Model file for the job. Use its own axes, mm. Face numbers are marked on the shaded views. Round coordinates to 2 decimals unless told otherwise and drop trailing zeros. Write each loop counter-clockwise with the first axis right and the second up, starting at its lowest first coordinate (ties: lowest second). Pieces come first, ordered by that corner, then holes. Notation, with made-up numbers: (-40, 71.5) - (-19, 71.5) arc R10 cw to (-19, 75.5) - close; hole circle Ø7 at (66, 28). An arc over 180 degrees is marked (long way). One line per item, written item: value.
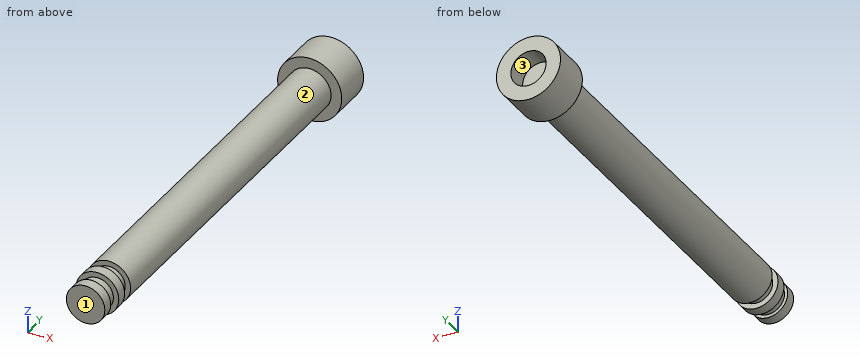
from build123d import *

# Parameters (mm, degrees)
SKETCH1_R           = 3
BOSS_EXTRUDE1_DEPTH = 3.7
SKETCH1_3_R         = 1.6
BOSS_EXTRUDE2_DEPTH = 1
SKETCH5_R           = 1.5
BOSS_EXTRUDE3_DEPTH = 35
SKETCH6_R           = 2
BOSS_EXTRUDE4_DEPTH = 1
SKETCH8_R           = 1.5
BOSS_EXTRUDE5_DEPTH = 2
SKETCH10_R          = 1.8
BOSS_EXTRUDE6_DEPTH = 1
SKETCH12_R          = 1.65
CUT_EXTRUDE1_DEPTH  = 2
SKETCH13_R          = 2
BOSS_EXTRUDE7_DEPTH = 34


with BuildPart() as part:
    # Sketch1 → Boss-Extrude1 (new body)
    with BuildSketch(Plane(origin=(0, 0, 0), x_dir=(1, 0, 0), z_dir=(0, 1, 0))):
        with Locations((-0.522013312, 0.511138034)):
            Circle(SKETCH1_R)
    extrude(amount=BOSS_EXTRUDE1_DEPTH)

    # Sketch1<3> → Boss-Extrude2 (add)
    with BuildSketch(Plane(origin=(0, 0, 0), x_dir=(1, 0, 0), z_dir=(0, 1, 0))):
        with Locations((-0.522013312, 0.511138034)):
            Circle(SKETCH1_3_R)
    extrude(amount=BOSS_EXTRUDE2_DEPTH)

    # Sketch5 → Boss-Extrude3 (add)
    with BuildSketch(Plane.XZ):
        with Locations((-0.522013312, -0.511138034)):
            Circle(SKETCH5_R)
    extrude(amount=BOSS_EXTRUDE3_DEPTH)

    # Sketch6 → Boss-Extrude4 (add)
    with BuildSketch(Plane.XZ.offset(35)):
        with Locations((-0.522013312, -0.511138034)):
            Circle(SKETCH6_R)
    extrude(amount=BOSS_EXTRUDE4_DEPTH)

    # Sketch8 → Boss-Extrude5 (add)
    with BuildSketch(Plane(origin=(0, -36, 0), x_dir=(-1, 0, 0), z_dir=(0, -1, 0))):
        with Locations((0.522013312, 0.511138034)):
            Circle(SKETCH8_R)
    extrude(amount=BOSS_EXTRUDE5_DEPTH)

    # Sketch10 → Boss-Extrude6 (add)
    with BuildSketch(Plane.XZ.offset(38)):
        with Locations((-0.522013312, -0.511138034)):
            Circle(SKETCH10_R)
    extrude(amount=-BOSS_EXTRUDE6_DEPTH)

    # Sketch12 → Cut-Extrude1 (cut)
    with BuildSketch(Plane(origin=(0, 3.7, 0), x_dir=(1, 0, 0), z_dir=(0, 1, 0))):
        with Locations((-0.522013312, 0.511138034)):
            Circle(SKETCH12_R)
    extrude(amount=-CUT_EXTRUDE1_DEPTH, mode=Mode.SUBTRACT)

    # Sketch13 → Boss-Extrude7 (add)
    with BuildSketch(Plane.XZ):
        with Locations((-0.522013312, -0.511138034)):
            Circle(SKETCH13_R)
    extrude(amount=BOSS_EXTRUDE7_DEPTH)


solid = part.part
1. Band-saw the part on B-B on x = -0.8. Write the cut outline in (y, z), plus the area to 3 significant figures.
Report:
outline: (-38, -2.29) - (-37, -2.29) - (-37, -1.99) - (-36, -1.99) - (-36, -2.49) - (-35, -2.49) - (-35, -1.99) - (-34, -1.99) - (-34, -2.49) - (0, -2.49) - (0, -3.5) - (3.7, -3.5) - (3.7, -2.14) - (1.7, -2.14) - (1.7, 1.12) - (3.7, 1.12) - (3.7, 2.48) - (0, 2.48) - (0, 1.47) - (-34, 1.47) - (-34, 0.96) - (-35, 0.96) - (-35, 1.47) - (-36, 1.47) - (-36, 0.96) - (-37, 0.96) - (-37, 1.27) - (-38, 1.27) - close
area: 164 mm²
2. Band-saw the part on A-A on z = -1.5. Write the cut outline in (x, y).
Report:
outline: (-3.35, 0) - (-2.26, 0) - (-2.26, -34) - (-1.65, -34) - (-1.65, -35) - (-2.26, -35) - (-2.26, -36) - (-1.65, -36) - (-1.65, -37) - (-2.03, -37) - (-2.03, -38) - (0.98, -38) - (0.98, -37) - (0.61, -37) - (0.61, -36) - (1.22, -36) - (1.22, -35) - (0.61, -35) - (0.61, -34) - (1.22, -34) - (1.22, 0) - (2.31, 0) - (2.31, 3.7) - (0.8, 3.7) - (0.8, 1.7) - (-1.84, 1.7) - (-1.84, 3.7) - (-3.35, 3.7) - close
3. Band-saw the part on D-D on x = 2. Write the cut outline in (y, z), plus the area to 3 significant figures.
Report:
outline: (0, -2.14) - (3.7, -2.14) - (3.7, 1.11) - (0, 1.11) - close
area: 12.0 mm²
4. Band-saw the part on C-C on y = 0.5. Write the cut outline in (x, z), plus the area to 3 significant figures.
Report:
outline: circle Ø6 at (-0.52, -0.51)
area: 28.3 mm²
5. Drop flat-ended pins along their axis: pin 1 (1.8 mm diameter, centred on x = -0.5, z = -1, fed in from +Y); pin 2 (2 mm diameter, centred on x = 1.5, y = -24, fed in from +Z); pin 3 (1 mm diameter, centred on x = 1.5, y = -31, fed in from +Z). Give the stop position or say it passes through.
Report:
pin 1: y = 1.7
pin 2: z = 1.21
pin 3: z = 0.79
6. Mould opens along Z. For the marked faces 1, 2 and 3 say: released by +Z, released by -Z, zero draft, split by the parting line, or undercut.
Report:
face 1: zero draft
face 2: split by the parting line
face 3: undercut
7. Wall check: probe 1 along Y at (x, z) = (-0.75, -2.1); probe 2 along Y at (x, z) = (-0.4, -2.25); probe 3 along Y at (x, z) = (1.4, -0.4). Give the ranges that are in metal, low to high. Write a range as [from, to].
Report:
probe 1: [-38, -37], [-36, -35], [-34, 1.7]
probe 2: [-38, -37], [-36, -35], [-34, 3.7]
probe 3: [-36, -35], [-34, 3.7]
